Design review of the part built by this model. Coordinates are the model's own, in mm. Face numbers are marked on the shaded views. A direction names the side the tool comes from. Coordinates: 2 decimals unless noted, no trailing zeros. Write each loop counter-clockwise with the first axis right and the second up, starting at its lowest first coordinate (ties: lowest second). Pieces come first, ordered by that corner, then holes. Notation, with made-up numbers: (-26, 78) - (-19, 78) arc R18 cw to (-19, 83) - close; hole circle Ø1 at (5.25, -2). An arc over 180 degrees is marked (long way). Use a Markdown table: item, result.
from build123d import *

# Parameters (mm, degrees)
F0_R     = 31.75
F0_R_2   = 19.05
F1_DEPTH = 38.1
F3_DEPTH = 15.875
F5_DEPTH = 6.35


with BuildPart() as f1:
    # F0 (on Top) → F1 (new body)
    with BuildSketch(Plane.XY):
        Circle(F0_R)
        Circle(F0_R_2, mode=Mode.SUBTRACT)
    extrude(amount=F1_DEPTH)

    # F2 (on face) → F3 (join)
    with BuildSketch(Plane(origin=(0, 0, 0), x_dir=(1, 0, 0), z_dir=(0, 0, -1))):
        with BuildLine():
            Line((-82.55, -25.4), (-19.05, -25.4))
            ThreePointArc((-19.05, -25.4), (-31.75, 0), (-19.05, 25.4))
            Line((-19.05, 25.4), (-82.55, 25.4))
            Line((-82.55, 25.4), (-82.55, -25.4))
        make_face()
    extrude(amount=-F3_DEPTH)

    # F4 (on Front) → F5 (join, symmetric)
    with BuildSketch(Plane.XZ):
        Polygon((-30.745536, 34.708899), (-50.8, 15.875), (-30.745536, 15.875), align=None)
    extrude(amount=F5_DEPTH, both=True)


solid = f1.part
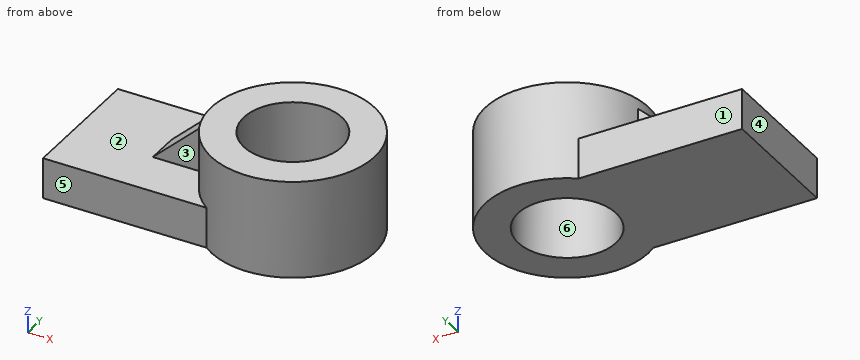
(1) Machinability: for the marked faces 1, 2 and 3, which of the approach directions +Z, -Z, +X, -X, +Y, -Y give a long, thin tool a straight path to every point of the face, cutting with its end or side? Answer none if there is none.
Determined:
| item | result |
|---|---|
| face 1 | +Z, -Z, -X, +Y |
| face 2 | +Z, -X |
| face 3 | +Z, -X, -Y |
(2) Take a section at D-D on y = 10. Write out the cut boundary in (x, z) (3 decimals).
Determined:
| item | result |
|---|---|
| outline | (-82.55, 0) - (-16.214, 0) - (-16.214, 38.1) - (-30.134, 38.1) - (-30.134, 15.875) - (-82.55, 15.875) - close; (16.214, 0) - (30.134, 0) - (30.134, 38.1) - (16.214, 38.1) - close |
(3) For L1, parallel to Y at x = 0, z = 16; L2, parallel to Z at x = -68.5, y = -10 (3 decimals); L3, parallel to Y at x = -75.5, z = 13.5, list the stretches that pass through material, from the lowest coordinate up. Write a range as from..to.
Determined:
| item | result |
|---|---|
| L1 | -31.75..-19.05, 19.05..31.75 |
| L2 | 0..15.875 |
| L3 | -25.4..25.4 |
(4) Draft analysis for pull direction Y (two halves, no side actions). For the marked faces 4, 5 and 6, state which applies: +Y half, -Y half, draft (parallel to the pull), parting line (faces both ways), or undercut.
Determined:
| item | result |
|---|---|
| face 4 | draft |
| face 5 | -Y half |
| face 6 | undercut |
(5) Take a section at B-B on y = 0. Write out the cut boundary in (x, z) (3 decimals).
Determined:
| item | result |
|---|---|
| outline | (-82.55, 0) - (-19.05, 0) - (-19.05, 38.1) - (-31.75, 38.1) - (-31.75, 33.766) - (-50.8, 15.875) - (-82.55, 15.875) - close; (19.05, 0) - (31.75, 0) - (31.75, 38.1) - (19.05, 38.1) - close |
(6) Take a section at C-C on z = 13.5. Write out the cut boundary in (x, y), and give its area (3 significant figures).
Determined:
| item | result |
|---|---|
| outline | (-82.55, -25.4) - (-19.05, -25.4) arc R31.75 ccw (long way) to (-19.05, 25.4) - (-82.55, 25.4) - close; hole circle Ø38.1 at (0, 0) |
| area | 4,800 mm2 |
(7) Take a section at A-A on x = 0. Write out the cut boundary in (y, z), and give its area (3 significant figures).
Determined:
| item | result |
|---|---|
| outline | (-31.75, 0) - (-19.05, 0) - (-19.05, 38.1) - (-31.75, 38.1) - close; (19.05, 0) - (31.75, 0) - (31.75, 38.1) - (19.05, 38.1) - close |
| area | 968 mm2 |
(8) For pin 1 (15 mm diameter, centred on x = -43.5, z = 25, fed in from -Y); pin 2 (8 mm diameter, centred on x = -38.5, z = 5, fed in from -Y); pin 3 (8 mm diameter, centred on y = -19.5, z = 13, fed in from +X), all flat-tipped, find the tip position at first contact; note any pin that passes through.
Determined:
| item | result |
|---|---|
| pin 1 | y = -6.35 |
| pin 2 | y = -25.4 |
| pin 3 | x = 27.71 |
